Geometry check sheet. Reference: the model listing, model coordinates, mm. Face numbers are marked on the shaded views. Give positions to 0.01 mm unless a question says otherwise; leave off trailing zeros. Order: outer loops, then holes, each group sorted by start corner. A loop starts at its lowest first (then second) coordinate and runs counter-clockwise, first axis right, second up. Notation, with made-up numbers: M -8,-18.5 L 10,-18.5 A17 ccw 10,-2.5 Z; hole C 52,3.25 d8. An arc over 180 degrees is marked long. Put each result on its own line as item: value. Start each with the question number.
Q1. Section check B-B on y = 0. Record the cut outline in (x, z), then the cut area to 4 significant figures.
Q2. Section check C-C on x = 2.9. Record the cut outline in (y, z), then the cut area to 3 significant figures.
Q3. Material ranges on L1, parallel to Y at x = 1.75, z = 2.5; L2, parallel to Z at x = 0.25, y = 1; L3, parallel to Y at x = 2.35, z = 1.5, recorded low to high.
Q4. Mould release check, pull along Z, two halves, no side actions. Record for the marked faces 1, 2 and 3: +Z half, -Z half, draft (parallel to the pull), parting line (faces both ways), or undercut.
Q5. Section check A-A on z = 2.5. Record the cut outline in (x, y), then the cut area to 3 significant figures.
Q6. Go/stop test with a flat-tipped pin: pin 1 (1.8 mm diameter, centred on y = 0, z = 2.5, fed in from -X). Record where the tip stops, or that it passes through.
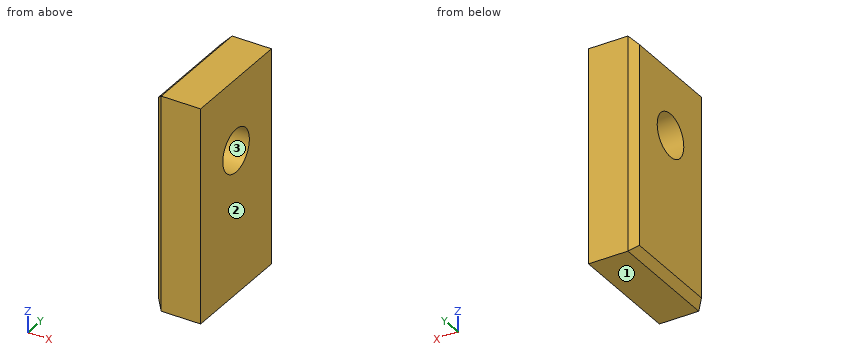
```python
from build123d import *

# Parameters (mm, degrees)
SKETCH_1_W          = 15
SKETCH_1_H          = 8
EXTRUDE_1_DEPTH     = 3.25
SKETCH_2_R          = 1.5
CUT_EXTRUDE_1_DEPTH = 10.100137362
CHAMFER_1_SIZE      = 0.5


with BuildPart() as part:
    # 草图1 → 凸台-拉伸1 (new body)
    with BuildSketch(Plane(origin=(0, 0, 0), x_dir=(0, 0, -1), z_dir=(1, 0, 0))):
        Rectangle(SKETCH_1_W, SKETCH_1_H)
    extrude(amount=EXTRUDE_1_DEPTH)

    # 草图2 → 切除-拉伸1 (cut, through all)
    with BuildSketch(Plane(origin=(3.25, 0, 0), x_dir=(0, 0, -1), z_dir=(1, 0, 0))):
        with Locations((-2.5, 0)):
            Circle(SKETCH_2_R)
    extrude(amount=-CUT_EXTRUDE_1_DEPTH, mode=Mode.SUBTRACT)

    # 倒角1
    chamfer_1_edges = [part.edges().sort_by_distance(p)[0] for p in [
        (0, 4, 0),
        (0, 0, -7.5),
        (0, -4, 0),
        (0, 0, 7.5),
    ]]
    chamfer(chamfer_1_edges, length=CHAMFER_1_SIZE)


solid = part.part
```
Results found:
1. outline: M 0,-7 L 0.5,-7.5 L 3.25,-7.5 L 3.25,1 L 0,1 Z; M 0,4 L 3.25,4 L 3.25,7.5 L 0.5,7.5 L 0,7 Z
1. area: 38.75 mm^2
2. outline: M -4,-7.5 L 4,-7.5 L 4,7.5 L -4,7.5 Z; hole C 0,2.5 d3
2. area: 113 mm^2
3. L1: y = -4 to -1.5, 1.5 to 4
3. L2: z = -7.25 to 1.38, 3.62 to 7.25
3. L3: y = -4 to -1.12, 1.12 to 4
4. face 1: -Z half
4. face 2: draft
4. face 3: undercut
5. outline: M 0,-3.5 L 0.5,-4 L 3.25,-4 L 3.25,-1.5 L 0,-1.5 Z; M 0,1.5 L 3.25,1.5 L 3.25,4 L 0.5,4 L 0,3.5 Z
5. area: 16.0 mm^2
6. pin 1: passes through
